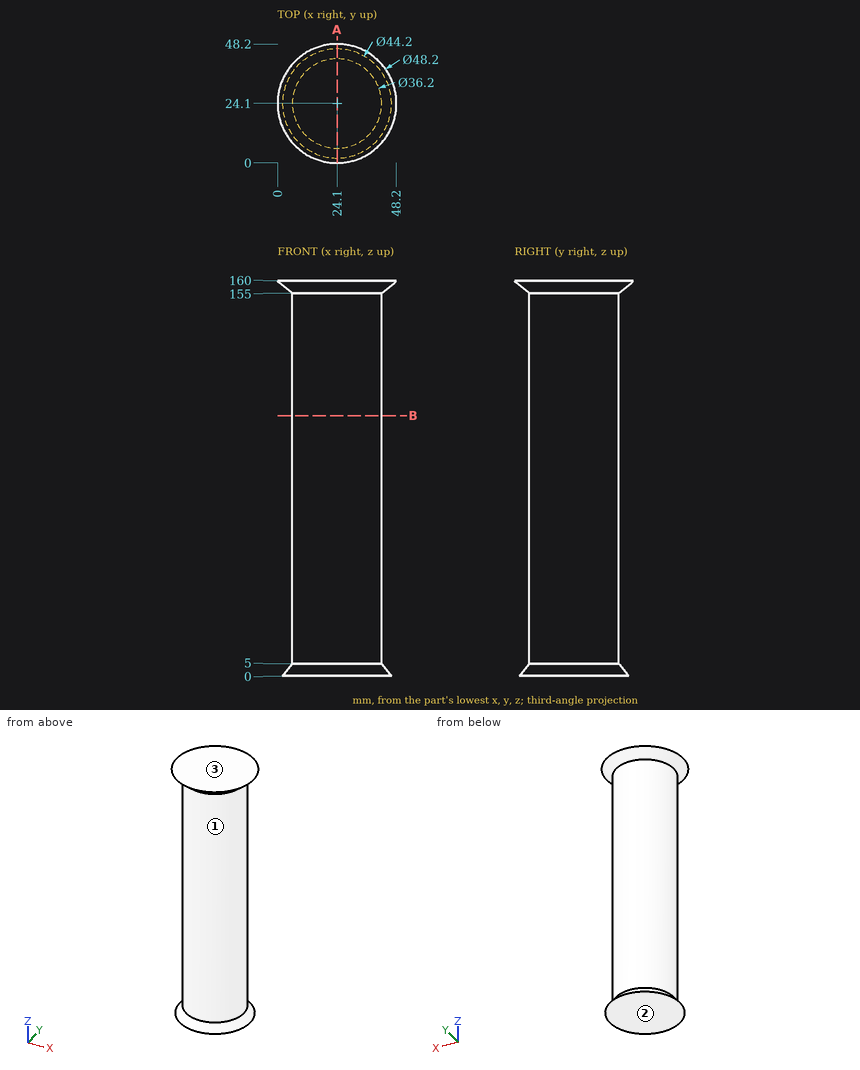
Geometry check sheet. Reference: drawing and pictorial views, mm from the part's lowest x, y, z. Coordinates: 2 decimals unless noted, no trailing zeros. Order: outer loops, then holes, each group sorted by start corner. A loop starts at its lowest first (then second) coordinate and runs counter-clockwise, first axis right, second up. Notation, with made-up numbers: (57, 89.5) - (73, 89.5) arc R26 ccw to (73, 108.5) - close; hole circle Ø11 at (-35.5, 44.5). An arc over 180 degrees is marked (long way). One line per item, written item: value.
(1) Sectioned sample at B-B (z = 105.5). Enter the section's corners in (x, y), and give its area (3 significant figures).
Data:
outline: circle Ø36.2 at (24.1, 24.1)
area: 1,030 mm^2
(2) Depth check by flat-ended pin: pin 1 Ø1 at (x, z) = (12.5, 124.5) entering from +Y; pin 2 Ø1.5 at (x, z) = (9, 76) entering from +Y; pin 3 Ø12 at (x, z) = (27.5, 81.5) entering from -Y. Enter the tip coordinate at first touch or a pass-through.
Data:
pin 1: stops at y = 38.4
pin 2: stops at y = 35.13
pin 3: stops at y = 6
(3) Release check for a two-part mould opening along Z. For the marked faces 1, 2 and 3 record: +Z half, -Z half, draft (parallel to the pull), parting line (faces both ways), or undercut.
Data:
face 1: undercut
face 2: -Z half
face 3: +Z half
(4) Sectioned sample at A-A (x = 24.1). Enter the section's corners in (y, z).
Data:
outline: (0, 160) - (6, 155) - (6, 5) - (2, 0) - (46.2, 0) - (42.2, 5) - (42.2, 155) - (48.2, 160) - close
(5) Thickness scan on probe 1 along Y at (x, z) = (23, 58.5); probe 2 along Z at (x, y) = (42, 14.5); probe 3 along Z at (x, y) = (30, 45). Record the ranges inside material, lowest first. Write a range as from..to.
Data:
probe 1: y = 6.03..42.17
probe 2: z = 0..2.24, 156.84..160
probe 3: z = 0..0.48, 158.01..160
